Geometry: final body of the model. Coordinates: model frame, mm. Face numbers are marked on the shaded views. A direction names the side the tool comes from. Give positions to 0.01 mm unless a question says otherwise; leave off trailing zeros. Write each loop counter-clockwise with the first axis right and the second up, starting at its lowest first coordinate (ties: lowest second). Pieces come first, ordered by that corner, then holes.
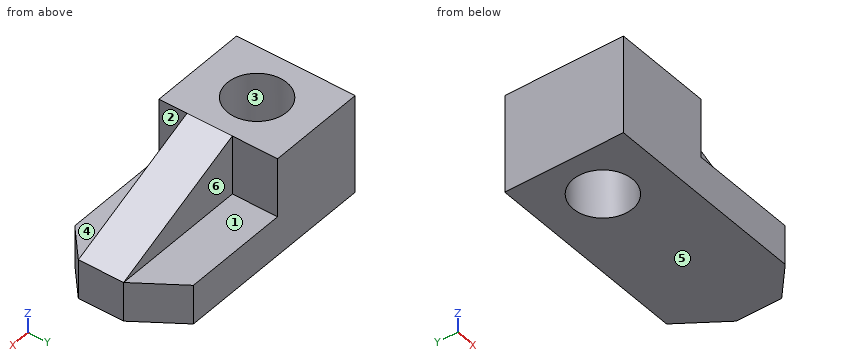
from build123d import *

# Parameters (mm, degrees)
F0_W      = 152.4
F0_H      = 76.2
F1_DEPTH  = 25.4
F2_W      = 63.5
F2_H      = 76.2
F3_DEPTH  = 38.1
F5_DEPTH  = 25.4
F7_DEPTH  = 25.4
F8_W      = 88.9
F8_H      = 29.105824
F9_DEPTH  = 38.1
F11_DEPTH = 38.1
F12_R     = 19.064579
F13_DEPTH = 76.2


with BuildPart() as f1:
    # F0 (on Top) → F1 (new body)
    with BuildSketch(Plane.XY):
        with Locations((1.330726, 9.390795)):
            Rectangle(F0_W, F0_H)
    extrude(amount=F1_DEPTH)

    # F2 (on face) → F3 (join)
    with BuildSketch(Plane.XY.offset(25.4)):
        with Locations((-43.119274, 9.390795)):
            Rectangle(F2_W, F2_H)
    extrude(amount=F3_DEPTH)

    # F4 (on face) → F5 (cut)
    with BuildSketch(Plane.XY.offset(25.4)):
        Polygon((57.543479, -28.709205), (77.530726, -28.709205), (77.530726, -10.720854), align=None)
    extrude(amount=-F5_DEPTH, mode=Mode.SUBTRACT)

    # F6 (on face) → F7 (cut)
    with BuildSketch(Plane.XY.offset(25.4)):
        Polygon((77.530726, 47.490795), (57.543479, 47.490795), (77.530726, 18.38497), align=None)
    extrude(amount=-F7_DEPTH, mode=Mode.SUBTRACT)

    # F8 (on face) → F9 (join)
    with BuildSketch(Plane.XY.offset(25.4)):
        with Locations((33.080726, 3.832058)):
            Rectangle(F8_W, F8_H)
    extrude(amount=F9_DEPTH)

    # F10 (on face) → F11 (cut)
    with BuildSketch(Plane.XZ.offset(10.720854)):
        Polygon((77.530726, 63.5), (-11.369274, 63.5), (77.530726, 25.4), align=None)
    extrude(amount=-F11_DEPTH, mode=Mode.SUBTRACT)

    # F12 (on face) → F13 (cut)
    with BuildSketch(Plane.XY.offset(63.5)):
        with Locations((-43.119274, 9.390795)):
            Circle(F12_R)
    extrude(amount=-F13_DEPTH, mode=Mode.SUBTRACT)


solid = f1.part
Q1. Section C-C on z = 47. Output: boundary loops of the cut face in (x, y).
Filled sheet:
outline: (-74.87, -28.71) - (-11.37, -28.71) - (-11.37, -10.72) - (27.13, -10.72) - (27.13, 18.38) - (-11.37, 18.38) - (-11.37, 47.49) - (-74.87, 47.49) - close; hole circle Ø38.13 at (-43.12, 9.39)
Q2. Pull-direction query (X, two-part tool) for the marked faces 1, 2 and 3; classes: released by +X, released by -X, zero draft, split by the parting line, or undercut.
Filled sheet:
face 1: zero draft
face 2: released by +X
face 3: undercut
Q3. Access query for the marked faces 4, 5 and 6. Directions: +Z, -Z, +X, -X, +Y, -Y. A direction counts if a zero-diameter tool reaches every point of the face in a straight line with its end or side. Return the directions, or none.
Filled sheet:
face 4: +Z, +X, -Y
face 5: -Z, +X, -X, +Y, -Y
face 6: +Z, +X, +Y
Q4. Section A-A on y = -6.5. Output: boundary loops of the cut face in (x, z), plus the area to 3 significant figures.
Filled sheet:
outline: (-74.87, 0) - (-53.65, 0) - (-53.65, 63.5) - (-74.87, 63.5) - close; (-32.59, 0) - (77.53, 0) - (77.53, 25.4) - (-11.37, 63.5) - (-32.59, 63.5) - close
area: 6,650 mm2
Q5. Section D-D on y = 33.5. Output: boundary loops of the cut face in (x, z).
Filled sheet:
outline: (-74.87, 0) - (67.15, 0) - (67.15, 25.4) - (-11.37, 25.4) - (-11.37, 63.5) - (-74.87, 63.5) - close
Q6. Pin query (flat end, axial travel): P1, Ø8.5, axis at y = 35.5, z = 50, coming from the +X side; P2, Ø23.5, axis at x = 46, y = 38, coming from the +Z side; P3, Ø19, axis at x = 12, z = 36.5, coming from the +Y side. Return the tip coordinate at first contact, or that it passes through.
Filled sheet:
P1: stops at x = -11.37
P2: stops at z = 25.4
P3: stops at y = 18.38
Q7. Ray query, line 1 along Z through (x, y) = (1, 44.5); line 2 along X through (y, z) = (42, 33.5); line 3 along Y through (x, z) = (54, 31). Return the intervals inside material, ascending.
Filled sheet:
line 1: z = 0 to 25.4
line 2: x = -74.87 to -11.37
line 3: y = -10.72 to 18.38
Q8. Section B-B on x = -53. Output: boundary loops of the cut face in (y, z).
Filled sheet:
outline: (-28.71, 0) - (-6.91, 0) - (-6.91, 63.5) - (-28.71, 63.5) - close; (25.7, 0) - (47.49, 0) - (47.49, 63.5) - (25.7, 63.5) - close
